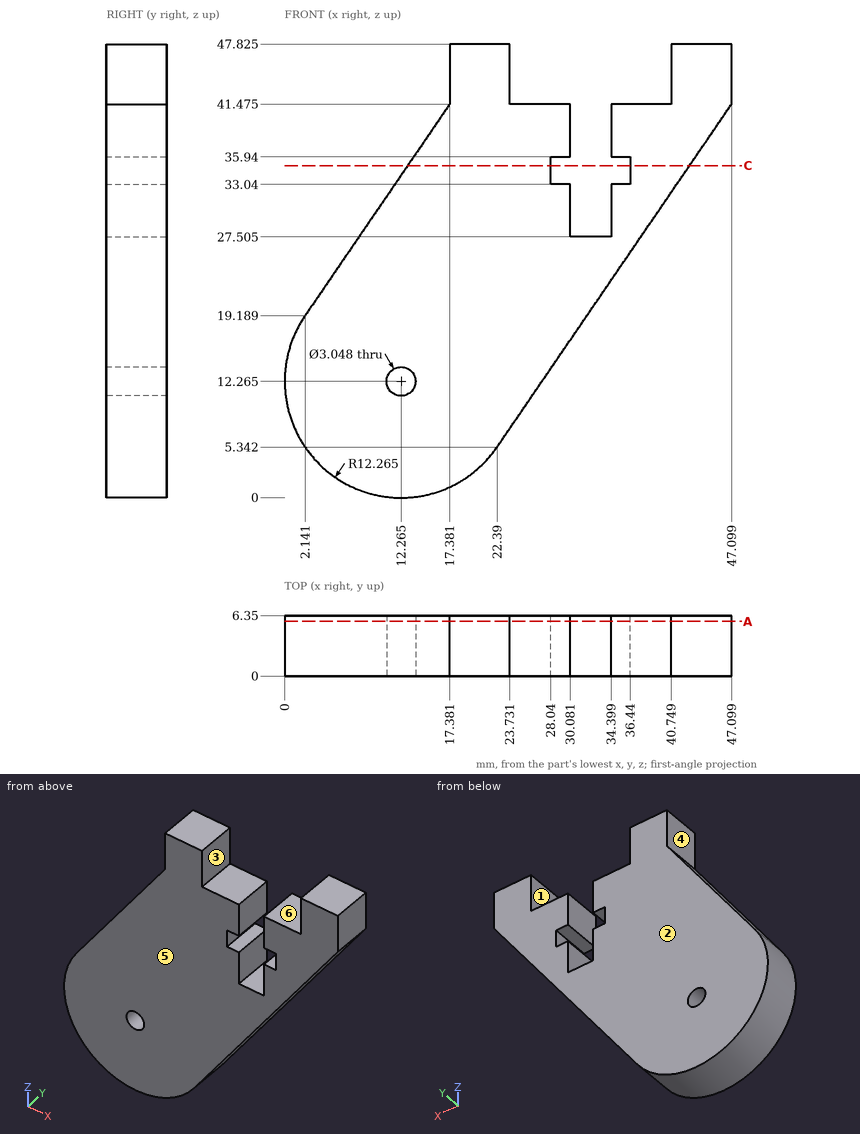
The drawing under review shows one solid part. Ordinate dimensions are in mm from its lowest x, y, z. A direction names the side the tool comes from. Coordinates: 2 decimals unless noted, no trailing zeros. Order: outer loops, then holes, each group sorted by start corner. A loop starts at its lowest first (then second) coordinate and runs counter-clockwise, first axis right, second up. Notation, with made-up numbers: (51.5, 51) -> (88.5, 51) arc R35 ccw to (88.5, 83) -> close; hole circle Ø5 at (62, 28.5). An arc over 180 degrees is marked (long way). Answer as CSV lines item,"result".
Q1. For the marked faces 1 and 2, list the 3-axis set-ups (+Z, -Z, +X, -X, +Y, -Y) from which the entire face can be reached by the end or side of a thin tool; tool diameter is ignored.
Model answer:
face 1,"+Z, +Y, -Y"
face 2,"+Z, -Z, +X, -X, +Y"
Q2. Clearance check with flat-ended pins moving along their axes: pin 1 Ø3 at (y, z) = (4, 8.5) entering from +X (1 decimal); pin 2 Ø2 at (x, y) = (35, 4.5) entering from -Z; pin 3 Ø0.6 at (x, y) = (29, 3.5) entering from +Z (1 decimal). State where each tip first meets the part, or that it passes through.
Model answer:
pin 1,"stops at x = 25.6"
pin 2,"stops at z = 22.32"
pin 3,"stops at z = 41.5"
Q3. Draft analysis for pull direction X (two halves, no side actions). For the marked faces 3, 4, 5 and 6, state which applies: released by +X, released by -X, zero draft, split by the parting line, or undercut.
Model answer:
face 3,"undercut"
face 4,"released by -X"
face 5,"zero draft"
face 6,"undercut"
Q4. Wall thickness on line 1 along X through (y, z) = (2, 43); line 2 along Z through (x, y) = (36, 4.5) (1 decimal); line 3 along X through (y, z) = (5.75, 30.5) (1 decimal): over which ranges is each line inside the solid? List them lowest first. Write a range as [from, to].
Model answer:
line 1,"x = [17.38, 23.73], [40.75, 47.1]"
line 2,"z = [25.2, 33], [35.9, 41.5]"
line 3,"x = [9.9, 30.1], [34.4, 39.6]"
Q5. We need section C-C (z = 35). State the section outline as (x, y) points.
Model answer:
outline,"(12.95, 0) -> (28.04, 0) -> (28.04, 6.35) -> (12.95, 6.35) -> close; (36.44, 0) -> (42.67, 0) -> (42.67, 6.35) -> (36.44, 6.35) -> close"
Q6. We need section A-A (y = 5.75). State the section outline as (x, z) points (1 decimal).
Model answer:
outline,"(2.1, 19.2) arc R12.3 ccw to (22.4, 5.3) -> (47.1, 41.5) -> (47.1, 47.8) -> (40.7, 47.8) -> (40.7, 41.5) -> (34.4, 41.5) -> (34.4, 35.9) -> (36.4, 35.9) -> (36.4, 33) -> (34.4, 33) -> (34.4, 27.5) -> (30.1, 27.5) -> (30.1, 33) -> (28, 33) -> (28, 35.9) -> (30.1, 35.9) -> (30.1, 41.5) -> (23.7, 41.5) -> (23.7, 47.8) -> (17.4, 47.8) -> (17.4, 41.5) -> close; hole circle Ø3 at (12.3, 12.3)"
